from build123d import *

# Parameters (mm, degrees)
SKETCH1_R           = 3.175
SKETCH1_W           = 25.4
SKETCH1_H           = 50.8
BOSS_EXTRUDE1_DEPTH = 3.175


with BuildPart() as part:
    # Sketch1 → Boss-Extrude1 (new body)
    with BuildSketch(Plane.XY):
        with BuildLine():
            Line((-392.019369126, 463.520831078), (-214.219369126, 463.520831078))
            ThreePointArc((-214.219369126, 463.520831078), (-205.239113005, 459.801087199), (-201.519369126, 450.820831078))
            Line((-201.519369126, 450.820831078), (-201.519369126, 323.820831078))
            ThreePointArc((-201.519369126, 323.820831078), (-205.239113005, 314.840574957), (-214.219369126, 311.120831078))
            Line((-214.219369126, 311.120831078), (-392.019369126, 311.120831078))
            ThreePointArc((-392.019369126, 311.120831078), (-400.999625247, 314.840574957), (-404.719369126, 323.820831078))
            Line((-404.719369126, 323.820831078), (-404.719369126, 450.820831078))
            ThreePointArc((-404.719369126, 450.820831078), (-400.999625247, 459.801087199), (-392.019369126, 463.520831078))
        make_face()
        with Locations((-239.619369126, 431.770831078)):
            Circle(SKETCH1_R, mode=Mode.SUBTRACT)
        with Locations((-239.619369126, 380.970831078)):
            Circle(SKETCH1_R, mode=Mode.SUBTRACT)
        with Locations((-265.019369126, 406.370831078)):
            Circle(SKETCH1_R, mode=Mode.SUBTRACT)
        with Locations((-366.619369126, 380.970831078)):
            Circle(SKETCH1_R, mode=Mode.SUBTRACT)
        with Locations((-341.219369126, 406.370831078)):
            Circle(SKETCH1_R, mode=Mode.SUBTRACT)
        with Locations((-366.619369126, 431.770831078)):
            Circle(SKETCH1_R, mode=Mode.SUBTRACT)
        with Locations((-265.019369126, 355.570831078)):
            Circle(SKETCH1_R, mode=Mode.SUBTRACT)
        with Locations((-341.219369126, 355.570831078)):
            Circle(SKETCH1_R, mode=Mode.SUBTRACT)
        with Locations((-303.119369126, 406.370831078)):
            Rectangle(SKETCH1_W, SKETCH1_H, mode=Mode.SUBTRACT)
    extrude(amount=BOSS_EXTRUDE1_DEPTH)


solid = part.part
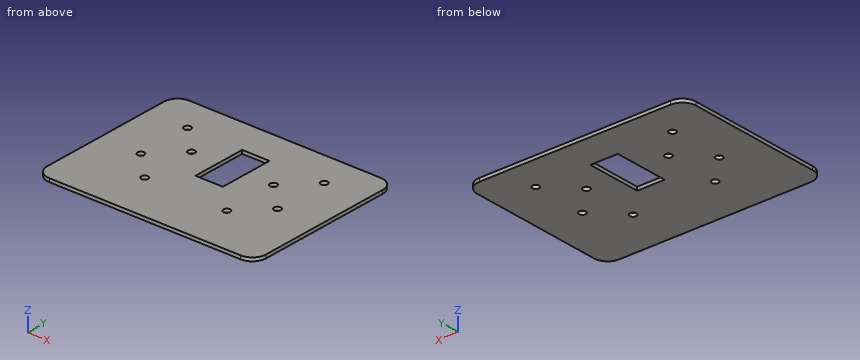
Input: part model. Units: mm. Frame: model coordinates. Coordinates: 2 decimals unless noted, no trailing zeros. Order: outer loops, then holes, each group sorted by start corner. A loop starts at its lowest first (then second) coordinate and runs counter-clockwise, first axis right, second up.
1. Ray query, line 1 along X through (y, z) = (416, 2.3); line 2 along Y through (x, z) = (-312.5, 0.25); line 3 along Y through (x, z) = (-211, 2.6). Return the intervals inside material, ascending.
Checked values:
line 1: x = -404.72 to -315.82, -290.42 to -201.52
line 2: y = 311.12 to 380.97, 431.77 to 463.52
line 3: y = 311.54 to 463.11
2. Cut plane D-D, the plane x = -265.5. Return loops of the section in (y, z) (3 decimals), plus the area to 3 significant figures.
Checked values:
outline: (311.121, 0) - (352.432, 0) - (352.432, 3.175) - (311.121, 3.175) - close; (358.709, 0) - (403.232, 0) - (403.232, 3.175) - (358.709, 3.175) - close; (409.509, 0) - (463.521, 0) - (463.521, 3.175) - (409.509, 3.175) - close
area: 444 mm2
3. Cut plane A-A, the plane y = 387.5. Return loops of the section in (x, z) (3 decimals).
Checked values:
outline: (-404.719, 0) - (-315.819, 0) - (-315.819, 3.175) - (-404.719, 3.175) - close; (-290.419, 0) - (-201.519, 0) - (-201.519, 3.175) - (-290.419, 3.175) - close
4. Cut plane C-C, the plane z = 0.9. Count the separate pieces of the cut face and the enclosed holes in it, plus the area to 3 significant figures.
Checked values:
separate pieces: 1
enclosed holes: 9
area: 29,300 mm2
5. Contact query for a flat-ended pin moving along its axis: P1, Ø4, axis at x = -366.62, y = 431.77, coming from the -Z side. Output: stop coordinate, or through.
Checked values:
P1: passes through
6. Cut plane B-B, the plane x = -305. Return loops of the section in (y, z) (3 decimals).
Checked values:
outline: (311.121, 0) - (380.971, 0) - (380.971, 3.175) - (311.121, 3.175) - close; (431.771, 0) - (463.521, 0) - (463.521, 3.175) - (431.771, 3.175) - close
